Answer from the drawing. Dimensions are ordinates in mm from the lowest x, y and z of the part. Coordinates: 2 decimals unless noted, no trailing zeros. Order: outer loops, then holes, each group sorted by start corner. A loop starts at its lowest first (then second) coordinate and runs counter-clockwise, first axis right, second up.
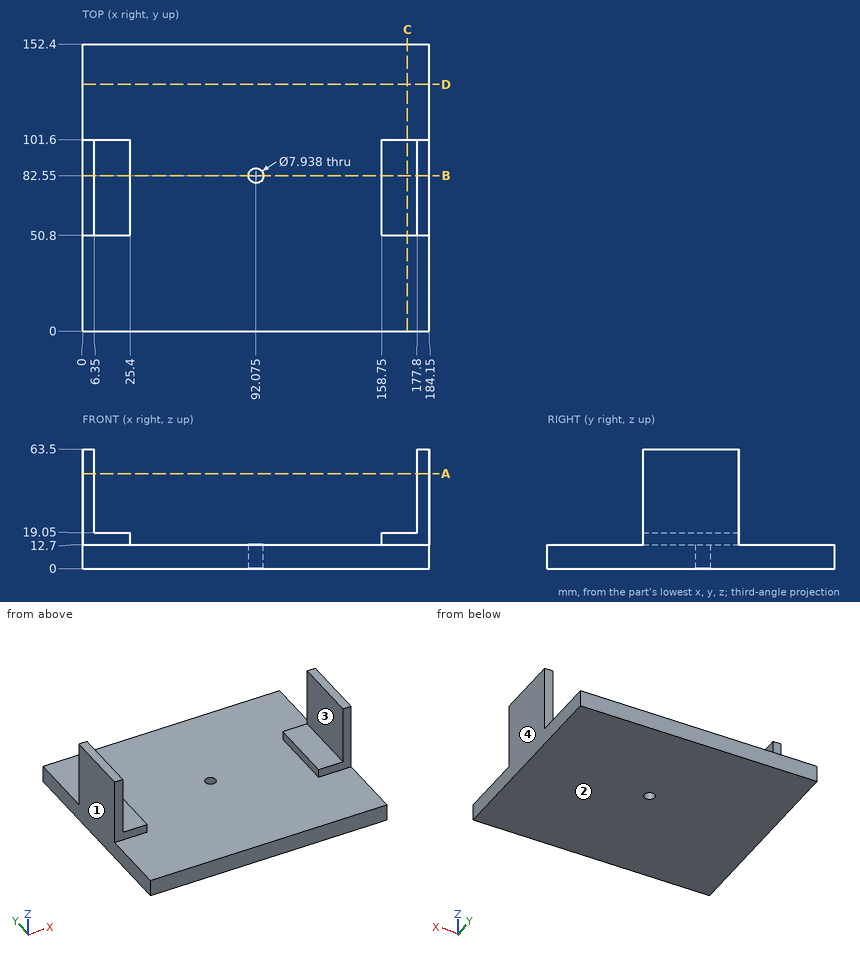
1. The part is cut by section D-D (y = 131). Determine the outline of the cut face in (x, z), plus the area to 3 significant figures.
2. Consider probe 1 along X at (y, z) = (51, 31.5); probe 2 along Y at (x, z) = (92, 12.5); probe 3 along Z at (x, y) = (118.5, 123). Determine where each line is inside the solid, lowest interval first.
3. Flat-ended cylindrical pins translate along their axes: pin 1 (9 mm diameter, centred on x = 92.075, y = 82.55, fed in from +Z); pin 2 (12.5 mm diameter, centred on x = 167, z = 46.5, fed in from -Y); pin 3 (21 mm diameter, centred on x = 18, y = 81.5, fed in from +Z). Find the tip coordinate at first contact, or state that the pin passes through.
4. The mould has two halves that part along X. Classify the marked faces 1, 2, 3 and 4: released by +X, released by -X, zero draft, split by the parting line, or undercut.
5. The part is cut by section A-A (z = 50.5). Determine the outline of the cut face in (x, y), plus the area to 3 significant figures.
6. The part is cut by section B-B (y = 82.55). Determine the outline of the cut face in (x, z).
7. The part is cut by section C-C (x = 172.5). Determine the outline of the cut face in (y, z), plus the area to 3 significant figures.
Worked out:
1. outline: (0, 0) - (184.15, 0) - (184.15, 12.7) - (0, 12.7) - close
1. area: 2,340 mm2
2. probe 1: x = 0 to 6.35, 177.8 to 184.15
2. probe 2: y = 0 to 78.58, 86.52 to 152.4
2. probe 3: z = 0 to 12.7
3. pin 1: stops at z = 12.7
3. pin 2: passes through
3. pin 3: stops at z = 19.05
4. face 1: released by -X
4. face 2: zero draft
4. face 3: undercut
4. face 4: released by +X
5. outline: (0, 50.8) - (6.35, 50.8) - (6.35, 101.6) - (0, 101.6) - close; (177.8, 50.8) - (184.15, 50.8) - (184.15, 101.6) - (177.8, 101.6) - close
5. area: 645 mm2
6. outline: (0, 0) - (88.11, 0) - (88.11, 12.7) - (25.4, 12.7) - (25.4, 19.05) - (6.35, 19.05) - (6.35, 63.5) - (0, 63.5) - close; (96.04, 0) - (184.15, 0) - (184.15, 63.5) - (177.8, 63.5) - (177.8, 19.05) - (158.75, 19.05) - (158.75, 12.7) - (96.04, 12.7) - close
7. outline: (0, 0) - (152.4, 0) - (152.4, 12.7) - (101.6, 12.7) - (101.6, 19.05) - (50.8, 19.05) - (50.8, 12.7) - (0, 12.7) - close
7. area: 2,260 mm2
